Autodesk Inventor part; units mm, degrees
ref_plane "YZ Plane" through (0, 0, 0) normal (1, 0, 0) x (0, 1, 0)
ref_plane "XZ Plane" through (0, 0, 0) normal (0, 1, 0) x (-1, 0, 0)
ref_plane "XY Plane" through (0, 0, 0) normal (0, 0, 1) x (1, 0, 0)
sketch "Sketch7" plane through (0, 0, 0) normal (0, 1, 0) x (-1, 0, 0)
  line L0 (12.7, 9.398) -> (-12.7, 9.398)
  line L1 (-12.7, 9.398) -> (-12.7, -9.398)
  line L2 (-12.7, -9.398) -> (12.7, -9.398)
  line L3 (12.7, -9.398) -> (12.7, 9.398)
  line L4 (12.7, 9.398) -> (-12.7, -9.398) construction
  line L5 (-12.7, 9.398) -> (12.7, -9.398) construction
  point P0 (0, 0)
  dimension "d53" = 18.796
  dimension "d54" = 25.4
extrude "Extrusion4" add sketch "Sketch7" along normal blind 63.5
sketch "Sketch8" plane through (0, 0, 0) normal (0, -1, 0) x (1, 0, 0)
  point P0 (0, 0)
  point P1 (0, 0)
hole "Hole7" at (0, 0, 0) direction (0, 1, 0) diameter 8.4328 depth 12.7
sketch "Sketch11" plane through (-12.7, 0, 9.398) normal (0, 0, 1) x (1, 0, 0)
  line L0 (12.7, 0) -> (12.7, 63.5) construction
  line L1 (0, 63.5) -> (25.4, 63.5) construction
  line L2 (19.05, 12.7) -> (19.05, 63.5)
  line L3 (19.05, 63.5) -> (6.35, 63.5)
  line L4 (6.35, 63.5) -> (6.35, 12.7)
  line L5 (6.35, 12.7) -> (19.05, 12.7)
  line L6 (19.05, 12.7) -> (6.35, 63.5) construction
  line L7 (19.05, 63.5) -> (6.35, 12.7) construction
  line L8 (0, 0) -> (25.4, 0)
  point P0 (12.7, 38.1)
  dimension "d85" = 12.7
  dimension "d86" = 50.8
  dimension "d87" = 12.7
extrude "Extrusion5" cut sketch "Sketch11" against normal through all
sketch "Sketch13" plane through (12.7, 0, 9.398) normal (1, 0, 0) x (0, 0, -1)
  line L0 (18.796, 63.5) -> (0, 63.5) construction
  line L1 (9.398, 63.5) -> (9.398, 0) construction
  point P0 (9.398, 53.975)
  dimension "d97" = 9.525
hole "Hole10" at (12.7, 53.975, 0) direction (-1, 0, 0) diameter 6.7564 end through all
properties part number "AngleBracketAttachementForDartActuator"
Input: part model. Units: mm. Frame: model coordinates. A direction names the side the tool comes from. Coordinates: 2 decimals unless noted, no trailing zeros. Loops run counter-clockwise (first coordinate to the right, second up) from the corner with the lowest first, then second, coordinate; pieces in that order, holes last. Notation, with made-up numbers: (63, 41) - (81, 41) arc R21 ccw to (81, 66) - close; hole circle Ø4 at (-32.75, 78.25). An arc over 180 degrees is marked (long way). Answer in a Markdown table with one row per item. Add a question column.
Item 1: Line query: line 1 along X through (y, z) = (15.5, -3.5); line 2 along Z through (x, y) = (0, 4.5); line 3 along X through (y, z) = (7.5, 0). Output: solid intervals per line, ascending. Write a range as [from, to].
Item 2: Access query for faces 4 (the cylindrical face through (9.481, 50.626, 0.44)), 5 (the flat face through (-2, 12.7, 4)). Directions: +Z, -Z, +X, -X, +Y, -Y. A direction counts if a zero-diameter tool reaches every point of the face in a straight line with its end or side. Return the directions, or none.
Item 3: Section query D-D on z = 6. Return the cut outline in (x, y).
Item 4: Section query A-A on x = 0. Return the cut outline in (y, z), then the cut area to 3 significant figures.
Item 5: Section query C-C on y = 29. Return the cut outline in (x, z).
Item 6: Mould query, pull axis Z, two halves, no side actions, for faces 1 (the cylindrical face through (-4.18, 6.44, 0.55)), 2 (the flat face through (10, 63.5, 0)), 3 (the flat face through (-8, 24, -9.398)). Classes: released by +Z, released by -Z, zero draft, split by the parting line, or undercut.
Item 7: Section query B-B on z = 0. Return the cut outline in (x, y).
Recorded:
| question | item | result |
|---|---|---|
| 1 | line 1 | [-12.7, -6.35], [6.35, 12.7] |
| 1 | line 2 | [-9.4, -4.22], [4.22, 9.4] |
| 1 | line 3 | [-12.7, -4.22], [4.22, 12.7] |
| 2 | face 4 | +X, -X |
| 2 | face 5 | +Z, -Z, +Y |
| 3 | outline | (-12.7, 0) - (12.7, 0) - (12.7, 63.5) - (6.35, 63.5) - (6.35, 12.7) - (-6.35, 12.7) - (-6.35, 63.5) - (-12.7, 63.5) - close |
| 4 | outline | (0, -9.4) - (12.7, -9.4) - (12.7, -4.22) - (0, -4.22) - close; (0, 4.22) - (12.7, 4.22) - (12.7, 9.4) - (0, 9.4) - close |
| 4 | area | 132 mm^2 |
| 5 | outline | (-12.7, -9.4) - (-6.35, -9.4) - (-6.35, 9.4) - (-12.7, 9.4) - close; (6.35, -9.4) - (12.7, -9.4) - (12.7, 9.4) - (6.35, 9.4) - close |
| 6 | face 1 | undercut |
| 6 | face 2 | zero draft |
| 6 | face 3 | released by -Z |
| 7 | outline | (-12.7, 0) - (-4.22, 0) - (-4.22, 12.7) - (-6.35, 12.7) - (-6.35, 50.6) - (-12.7, 50.6) - close; (-12.7, 57.35) - (-6.35, 57.35) - (-6.35, 63.5) - (-12.7, 63.5) - close; (4.22, 0) - (12.7, 0) - (12.7, 50.6) - (6.35, 50.6) - (6.35, 12.7) - (4.22, 12.7) - close; (6.35, 57.35) - (12.7, 57.35) - (12.7, 63.5) - (6.35, 63.5) - close |
